from build123d import *

# Parameters (mm, degrees)
F1_DEPTH = 25


with BuildPart() as f1:
    # F0 (on Front) → F1 (new body)
    with BuildSketch(Plane.XZ):
        with BuildLine():
            ThreePointArc((0, 5), (3.535534, 3.535534), (5, 0))
            ThreePointArc((5, 0), (4.924039, -0.868241), (4.698463, -1.710101))
            Line((4.698463, -1.710101), (1.120615, -11.540158))
            ThreePointArc((1.120615, -11.540158), (2.017935, -13.966481), (4.558306, -13.477866))
            Line((4.558306, -13.477866), (9.349836, -7.522006))
            ThreePointArc((9.349836, -7.522006), (11.318084, -3.987604), (12, 0))
            Line((12, 0), (12, 30))
            ThreePointArc((12, 30), (10.174311, 31.992389), (8.030384, 30.347296))
            Line((8.030384, 30.347296), (5.548481, 16.271721))
            ThreePointArc((5.548481, 16.271721), (4.695037, 14.959451), (3.157822, 14.663838))
            ThreePointArc((3.157822, 14.663838), (1.587832, 14.915723), (0, 15))
            Line((0, 15), (0, 5))
        make_face()
    extrude(amount=F1_DEPTH)

    # F2: F1 across face


with BuildPart() as f1_1:
    add(f1.part)
    add(f1.part.mirror(Plane(origin=(0, -12.5, 10), x_dir=(0, -1, 0), z_dir=(-1, 0, 0))))


solid = f1_1.part
Input: part model. Units: mm. Frame: model coordinates. A direction names the side the tool comes from. Round coordinates to 2 decimals unless told otherwise and drop trailing zeros. Loops run counter-clockwise (first coordinate to the right, second up) from the corner with the lowest first, then second, coordinate; pieces in that order, holes last. Notation, with made-up numbers: (-6, 17) -> (24, 17) arc R8 cw to (24, 22) -> close; hole circle Ø5 at (56.25, -4.75). An arc over 180 degrees is marked (long way). Answer as a JSON object with one key per item and string values. Group by question number.
1) Reachability of faces 4 (the cylindrical face through (-4.926, -12.325, -0.856)), 5 (the flat face through (-6.807, -12.325, 23.408)), 6 (the flat face through (0, -25, 9)) from +Z, -Z, +X, -X, +Y, -Y: full face, straight path, thin tool, end or side. Return the list, or none.
2) Draft query along X for faces 1 (the cylindrical face through (10, -12, 32)), 2 (the cylindrical face through (-11.3, -12.32, -4.04)), 3 (the cylindrical face through (11.3, -12.32, -4.04)). Return one class per face: +X half, -X half, draft (parallel to the pull), parting line (faces both ways), or undercut.
3) Section query A-A on z = 18. Output: boundary loops of the cut face in (x, y), plus the area to 3 significant figures.
4) Section query C-C on z = 4.5. Output: boundary loops of the cut face in (x, y).
5) Pin query (flat end, axial travel): pin 1 (1 mm diameter, centred on x = -4, y = -2.5, fed in from +Z); pin 2 (1 mm diameter, centred on x = -9, y = -5, fed in from -Z); pin 3 (1 mm diameter, centred on x = 5, y = -7.5, fed in from -Z). Return the tip coordinate at first contact, or that it passes through.
6) Ray query, L1, parallel to X at y = -17.25, z = -8.5; L2, parallel to X at y = -16, z = -11.5; L3, parallel to Z at x = -0.5, y = -23. Return the intervals inside material, ascending.
7) Section query B-B on y = -22. Output: boundary loops of the cut face in (x, z).
8) Section query D-D on x = -10. Output: boundary loops of the cut face in (y, z).
Reply:
{
 "1": {"face 4": "+Y, -Y", "face 5": "+Z, +Y, -Y", "face 6": "+Z, -Z, +X, -X, -Y"},
 "2": {"face 1": "undercut", "face 2": "-X half", "face 3": "+X half"},
 "3": {"outline": "(-12, -25) -> (-5.85, -25) -> (-5.85, 0) -> (-12, 0) -> close; (5.85, -25) -> (12, -25) -> (12, 0) -> (5.85, 0) -> close", "area": "307 mm2"},
 "4": {"outline": "(-12, -25) -> (-2.18, -25) -> (-2.18, 0) -> (-12, 0) -> close; (2.18, -25) -> (12, -25) -> (12, 0) -> (2.18, 0) -> close"},
 "5": {"pin 1": "stops at z = 14.84", "pin 2": "stops at z = -8.58", "pin 3": "stops at z = -13.55"},
 "6": {"L1": "x = -8.56 to -2.23, 2.23 to 8.56", "L2": "x = -6.15 to -1.14, 1.14 to 6.15", "L3": "z = 4.97 to 14.99"},
 "7": {"outline": "(-12, 0) arc R12 ccw to (-9.35, -7.52) -> (-4.56, -13.48) arc R2 ccw to (-1.12, -11.54) -> (-4.7, -1.71) arc R5 cw to (-5, 0) arc R5 cw to (5, 0) arc R5 cw to (4.7, -1.71) -> (1.12, -11.54) arc R2 ccw to (4.56, -13.48) -> (9.35, -7.52) arc R12 ccw to (12, 0) -> (12, 30) arc R2 ccw to (8.03, 30.35) -> (5.55, 16.27) arc R2 cw to (3.16, 14.66) arc R15 ccw to (0, 15) arc R15 ccw to (-3.16, 14.66) arc R2 cw to (-5.55, 16.27) -> (-8.03, 30.35) arc R2 ccw to (-12, 30) -> close"},
 "8": {"outline": "(-25, -6.63) -> (0, -6.63) -> (0, 32) -> (-25, 32) -> close"}
}
